Geometry check sheet. Reference: the model listing, model coordinates, mm. A direction names the side the tool comes from. Coordinates: 2 decimals unless noted, no trailing zeros. Loops run counter-clockwise (first coordinate to the right, second up) from the corner with the lowest first, then second, coordinate; pieces in that order, holes last. Notation, with made-up numbers: (3, 51.25) - (61, 51.25) arc R21 ccw to (61, 66.25) - close; hole circle Ø5 at (55, -8.5). An arc over 180 degrees is marked (long way). Write item = value, one per line. Start each with the question number.
from build123d import *

# Parameters (mm, degrees)
F1_DEPTH = 70
F2_DEPTH = 30
F4_DEPTH = 30


with BuildPart() as f1:
    # F0 (on Front) → F1 (new body)
    with BuildSketch(Plane.XZ):
        with BuildLine():
            Line((0, 2), (0, 5))
            ThreePointArc((0, 5), (-3.535534, -3.535534), (5, 0))
            ThreePointArc((5, 0), (4.894532, 1.021548), (4.582576, 2))
            Line((4.582576, 2), (0, 2))
        make_face()
        with BuildLine():
            ThreePointArc((4.582576, 2), (2.738613, 4.1833), (0, 5))
            Line((0, 5), (0, 2))
            Line((0, 2), (4.582576, 2))
        make_face()
    extrude(amount=F1_DEPTH)

    # F0 (on Front) → F2 (join)
    with BuildSketch(Plane.XZ):
        with BuildLine():
            Line((12, 5), (0, 5))
            ThreePointArc((0, 5), (2.738613, 4.1833), (4.582576, 2))
            Line((4.582576, 2), (9, 2))
            ThreePointArc((9, 2), (11.12132, 1.12132), (12, -1))
            Line((12, -1), (12, -25))
            Line((12, -25), (15, -25))
            Line((15, -25), (15, -3))
            Line((15, -3), (15, 2))
            ThreePointArc((15, 2), (14.12132, 4.12132), (12, 5))
        make_face()
    extrude(amount=F2_DEPTH)

    # F3 (on face) → F4 (join)
    with BuildSketch(Plane.XZ.offset(70)):
        with BuildLine():
            ThreePointArc((0, -5), (-2.738613, -4.1833), (-4.582576, -2))
            Line((-4.582576, -2), (-50, -2))
            Line((-50, -2), (-50, -5))
            Line((-50, -5), (0, -5))
        make_face()
    extrude(amount=-F4_DEPTH)


solid = f1.part
(1) Depth check by flat-ended pin: pin 1 (2.5 mm diameter, centred on x = -35.5, z = -3.5, fed in from +Y); pin 2 (5 mm diameter, centred on y = -20.5, z = -3, fed in from -X); pin 3 (15 mm diameter, centred on x = -25, y = -57.5, fed in from +Z). Enter the tip coordinate at first touch or a pass-through.
(2) Draft check along X on faces 1 (the face through (11.1, -14.79, 1.14)), 2 (the face through (-27, -55, -2)), 3 (the face through (14.14, -14.79, 4.1)). Enter one of: pulls with the +X half, pulls with the -X half, needs draft (parallel to the pull), parting line crosses it, or undercut.
(3) Sectioned sample at C-C on z = -14.75. Enter the section's corners in (x, y), plus the area to 3 significant figures.
(4) Sectioned sample at A-A on y = -22. Enter the section's corners in (x, z), plus the area to 3 significant figures.
(5) Sectioned sample at B-B on x = -19. Enter the section's corners in (y, z), plus the area to 3 significant figures.
(6) Tool access check on faces 4 (the face through (12, -15, -13)), 5 (the face through (15, -15, -12)). Record the directions out of +Z, -Z, +X, -X, +Y, -Y that give a thin tool (end or side, any length) a straight path to the whole face; none if there is none.
(7) Scan lines: line 1 (X direction, y = -20, z = -8); line 2 (Y direction, x = -37, z = -4); line 3 (X direction, y = -4, z = -2.75). Record each from-to range of solid material in increasing order.
Working result:
q1.pin_1 = -40
q1.pin_2 = -4.97
q1.pin_3 = -2
q2.face_1 = undercut
q2.face_2 = needs draft
q2.face_3 = pulls with the +X half
q3.outline = (12, -30) - (15, -30) - (15, 0) - (12, 0) - close
q3.area = 90.0 mm2
q4.outline = (0, 5) arc R5 ccw (long way) to (5, 0) arc R5 ccw to (4.58, 2) - (9, 2) arc R3 cw to (12, -1) - (12, -25) - (15, -25) - (15, 2) arc R3 ccw to (12, 5) - close
q4.area = 195 mm2
q5.outline = (-70, -5) - (-40, -5) - (-40, -2) - (-70, -2) - close
q5.area = 90.0 mm2
q6.face_4 = -Z, +Y, -Y
q6.face_5 = +Z, -Z, +X, +Y, -Y
q7.line_1 = 12 to 15
q7.line_2 = -70 to -40
q7.line_3 = -4.18 to 4.18, 12 to 15
